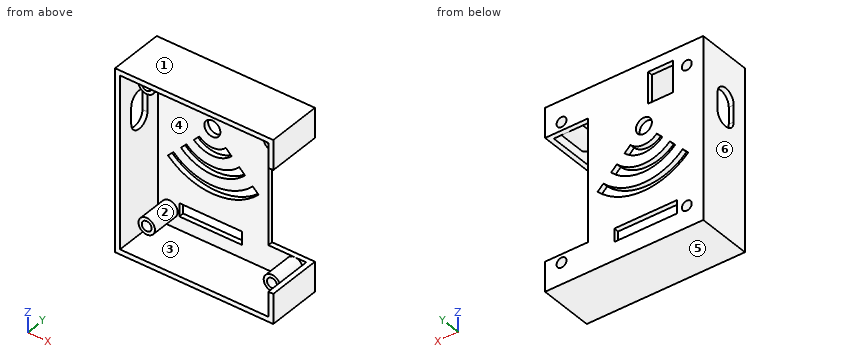
Autodesk Inventor part; units mm, degrees
ref_plane "YZ Plane" through (0, 0, 0) normal (1, 0, 0) x (0, 1, 0)
ref_plane "XZ Plane" through (0, 0, 0) normal (0, 1, 0) x (-1, 0, 0)
ref_plane "XY Plane" through (0, 0, 0) normal (0, 0, 1) x (1, 0, 0)
sketch "Sketch1" plane through (0, 0, 0) normal (0, 1, 0) x (-1, 0, 0)
  point P0 (0, 0)
sketch "Sketch2" plane through (0, 0, 0) normal (0, 1, 0) x (-1, 0, 0)
  line L0 (-24, 27.5) -> (24, 27.5)
  line L1 (24, 27.5) -> (24, -27.5)
  line L2 (24, -27.5) -> (-24, -27.5)
  line L3 (-24, -27.5) -> (-24, 27.5)
  line L4 (22.5, 26) -> (-22.5, 26)
  line L5 (-22.5, 26) -> (-22.5, -26)
  line L6 (-22.5, -26) -> (22.5, -26)
  line L7 (22.5, -26) -> (22.5, 26)
  dimension "d1" = 55
extrude "Extrusion1" add sketch "Sketch2" along normal blind 6
sketch "Sketch3" plane through (0, 6, 0) normal (0, 1, 0) x (1, 0, 0)
  circle A0 centre (19, -21) radius 2.5
  circle A1 centre (-19, -21) radius 2.5
  circle A2 centre (-19, 21) radius 2.5
  circle A3 centre (19, 21) radius 2.5
  circle A4 centre (-19, -21) radius 1.5
  circle A5 centre (-19, 21) radius 1.5
  circle A6 centre (19, 21) radius 1.5
  circle A7 centre (19, -21) radius 1.5
  line L0 (-22.5, -26) -> (22.5, -26)
  line L1 (22.5, -26) -> (22.5, 26)
  line L2 (22.5, 26) -> (-22.5, 26)
  line L3 (-22.5, 26) -> (-22.5, -26)
  line L4 (-24, -27.5) -> (24, -27.5)
  line L5 (24, -27.5) -> (24, 27.5)
  line L6 (24, 27.5) -> (-24, 27.5)
  line L7 (-24, 27.5) -> (-24, -27.5)
  dimension "d16" = 3
  dimension "d17" = 3
  dimension "d18" = 3
extrude "Extrusion2" add sketch "Sketch3" along normal blind 9
sketch "Sketch4" plane through (24, 0, 27.5) normal (1, 0, 0) x (0, 0, -1)
  line L0 (9, 6) -> (9, 15)
  line L1 (9, 15) -> (46, 15)
  line L2 (55, 0) -> (0, 0)
  line L3 (46, 6) -> (46, 15)
  line L4 (46, 15) -> (9, 15)
  line L5 (9, 15) -> (9, 6)
  line L6 (9, 0) -> (46, 0)
  line L7 (46, 0) -> (46, 15)
  line L8 (46, 15) -> (9, 15)
  line L9 (9, 15) -> (9, 0)
  point P0 (27.5, 0)
extrude "Extrusion3" cut sketch "Sketch4" against normal up to surface (1.5 mm away)
sketch "Sketch5" plane through (0, 15, 0) normal (0, 1, 0) x (1, 0, 0)
  line L0 (-24, -27.5) -> (24, -27.5)
  line L1 (-24, 27.5) -> (-24, -27.5)
  line L2 (24, -27.5) -> (-24, -27.5)
  line L3 (-24, -27.5) -> (-24, 27.5)
  line L4 (-24, 27.5) -> (24, 27.5)
  line L5 (22.5, -18.5) -> (24, -18.5)
  line L6 (24, -18.5) -> (11, -18.5)
  line L7 (24, 18.5) -> (24, 27.5)
  line L8 (24, 18.5) -> (11, 18.5)
  line L9 (11, 18.5) -> (11, -18.5)
  line L10 (24, 27.5) -> (24, 18.5)
  line L11 (24, -18.5) -> (24, -27.5)
  circle A0 centre (-19, -21) radius 1.5
  circle A1 centre (-19, -21) radius 1.5
  circle A2 centre (-19, 21) radius 1.5
  circle A3 centre (-19, 21) radius 1.5
  circle A4 centre (19, 21) radius 1.5
  circle A5 centre (19, 21) radius 1.5
  circle A6 centre (19, -21) radius 1.5
  circle A7 centre (19, -21) radius 1.5
  point P0 (0, 0)
extrude "Extrusion4" add sketch "Sketch5" along normal blind 1.5
sketch "Sketch6" plane through (-24, 0, -27.5) normal (-1, 0, 0) x (0, 0, 1)
  line L0 (41.4364, 10.844) -> (36.321, 10.844)
  line L1 (36.321, 4.444) -> (41.4364, 4.444)
  arc A0 (41.4364, 4.444) -> (41.4364, 10.844) centre (41.4364, 7.644) ccw
  arc A1 (36.321, 10.844) -> (36.321, 4.444) centre (36.321, 7.644) ccw
  point P0 (27.5, 0)
extrude "Extrusion5" cut sketch "Sketch6" against normal up to surface (1.5 mm away)
sketch "Sketch7" plane through (0, 16.5, 0) normal (0, 1, 0) x (1, 0, 0)
  circle A0 centre (-19, 21) radius 1.5
  line L0 (3, 18) -> (-16, 18)
  line L1 (-16, 18) -> (-16, 22)
  line L2 (-16, 22) -> (3, 22)
  line L3 (3, 22) -> (3, 18)
  point P0 (0, 0)
  dimension "d37" = 19
  dimension "d38" = 4
extrude "Extrusion6" cut sketch "Sketch7" against normal through all contours L0 L1 L2 L3
sketch "Sketch8" plane through (0, 16.5, 0) normal (0, 1, 0) x (1, 0, 0)
  line L0 (-14.75, -24.25) -> (-7.25, -24.25)
  line L1 (-7.25, -24.25) -> (-7.25, -14.75)
  line L2 (-7.25, -14.75) -> (-14.75, -14.75)
  line L3 (-14.75, -14.75) -> (-14.75, -24.25)
  point P0 (0, 0)
  dimension "d44" = 7.5
  dimension "d45" = 9.5
extrude "Extrusion7" cut sketch "Sketch8" against normal through all
sketch "Sketch9" plane through (0, 16.5, 0) normal (0, 1, 0) x (1, 0, 0)
  circle A0 centre (-5.9739, -8.7344) radius 2.43
  arc A1 (-1.887, -4.8042) -> (-9.9041, -4.6475) centre (-5.9739, -8.7344) ccw
  arc A2 (-0.1355, -3.1199) -> (-11.5884, -2.8959) centre (-5.9739, -8.7344) ccw
  arc A3 (2.1999, -0.874) -> (-13.8342, -0.5606) centre (-5.9739, -8.7344) ccw
  arc A4 (3.9514, 0.8103) -> (-15.5186, 1.1909) centre (-5.9739, -8.7344) ccw
  arc A5 (6.2868, 3.0561) -> (-17.7644, 3.5263) centre (-5.9739, -8.7344) ccw
  arc A6 (8.0389, 4.741) -> (-19.3203, 5.4014) centre (-5.9739, -8.7344) ccw
  line L0 (-19.3203, 5.4014) -> (-19.4487, 5.2778)
  line L1 (-19.4487, 5.2778) -> (-19.3445, 5.1695)
  line L2 (-17.7644, 3.5263) -> (-19.3445, 5.1695)
  line L3 (-13.8342, -0.5606) -> (-15.5186, 1.1909)
  line L4 (-9.9041, -4.6475) -> (-11.5884, -2.8959)
  line L5 (-1.887, -4.8042) -> (-0.1355, -3.1199)
  line L6 (2.1999, -0.874) -> (3.9514, 0.8103)
  line L7 (6.2868, 3.0561) -> (8.0389, 4.741)
  point P0 (0, 0)
  dimension "d48" = 4.86
extrude "Extrusion8" cut sketch "Sketch9" against normal through all
properties part number "Box2_Top"
Part model, mm, in its own coordinate system. Face numbers are marked on the shaded views. A direction names the side the tool comes from. Give positions to 0.01 mm unless a question says otherwise; leave off trailing zeros. Write each loop counter-clockwise with the first axis right and the second up, starting at its lowest first coordinate (ties: lowest second). Pieces come first, ordered by that corner, then holes. Notation, with made-up numbers: (83.25, 81.5) -> (126.25, 81.5) arc R29 ccw to (126.25, 106.5) -> close; hole circle Ø2 at (-9.75, 17.5). An arc over 180 degrees is marked (long way). Put each result on its own line as item: value. Start each with the question number.
Item 1: Cut at D-D (z = 8). List the corners of the cut face in (x, y).
Item 2: Pull direction Z, two halves, no side cores. Call the marked faces 3, 4, 5 and 6: pulls with the +Z half, pulls with the -Z half, needs draft (parallel to the pull), parting line crosses it, or undercut.
Item 3: Which spindle directions (+Z, -Z, +X, -X, +Y, -Y) get a long thin tool onto all of the face, cutting with end or side? Do the marked faces 1 and 2. Say none if no direction does.
Item 4: Cut at B-B (z = -21). List the corners of the cut face in (x, y).
Item 5: Cut at A-A (y = 13.25). State how many separate pieces and enclosed holes the cut face has, then the cut area to 3 significant figures.
Item 6: Pin check, flat tips, straight feed: pin 1 Ø5 at (x, z) = (-19, 21) entering from -Y; pin 2 Ø0.8 at (y, z) = (15.5, -1) entering from +X; pin 3 Ø22.5 at (x, z) = (7.5, 2.5) entering from -Y. Stop position of each tip, or through.
Item 7: Wall check: L1, parallel to Z at x = -19, y = 8; L2, parallel to X at y = 11, z = 21; L3, parallel to Z at x = -3, y = 11. Give the ranges that are in metal, low to high. Write a range as [from, to].
Item 8: Cut at C-C (x = -2.5). List the corners of the cut face in (y, z), then the cut area to 3 significant figures.
Answer list:
1. outline: (-24, 0) -> (-22.5, 0) -> (-22.5, 4.55) -> (-24, 4.55) -> close; (-24, 10.74) -> (-22.5, 10.74) -> (-22.5, 15) -> (-8.29, 15) -> (-8.29, 16.5) -> (-24, 16.5) -> close; (-3.66, 15) -> (11, 15) -> (11, 16.5) -> (-3.66, 16.5) -> close
2. face 3: undercut
2. face 4: undercut
2. face 5: pulls with the -Z half
2. face 6: needs draft
3. face 1: +Z, +X, -X, +Y, -Y
3. face 2: -Y
4. outline: (-24, 0) -> (-22.5, 0) -> (-22.5, 15) -> (-21.5, 15) -> (-21.5, 6) -> (-20.5, 6) -> (-20.5, 16.5) -> (-24, 16.5) -> close; (-17.5, 6) -> (-16.5, 6) -> (-16.5, 15) -> (-16, 15) -> (-16, 16.5) -> (-17.5, 16.5) -> close; (3, 15) -> (16.5, 15) -> (16.5, 6) -> (17.5, 6) -> (17.5, 16.5) -> (3, 16.5) -> close; (20.5, 6) -> (21.5, 6) -> (21.5, 15) -> (22.5, 15) -> (22.5, 0) -> (24, 0) -> (24, 16.5) -> (20.5, 16.5) -> close
5. separate pieces: 5
5. enclosed holes: 4
5. area: 295 mm2
6. pin 1: stops at y = 6
6. pin 2: stops at x = 11
6. pin 3: stops at y = 15
7. L1: z = [-27.5, -26], [-23.5, -22.5], [-19.5, -18.5], [18.5, 19.5], [22.5, 23.5], [26, 27.5]
7. L2: x = [-24, -22.5], [-21.5, -20.5], [-17.5, -16.5], [16.5, 17.5], [20.5, 21.5], [22.5, 24]
7. L3: z = [-27.5, -26], [26, 27.5]
8. outline: (0, -27.5) -> (16.5, -27.5) -> (16.5, -22) -> (15, -22) -> (15, -26) -> (0, -26) -> close; (0, 26) -> (15, 26) -> (15, 4.25) -> (16.5, 4.25) -> (16.5, 27.5) -> (0, 27.5) -> close; (15, -18) -> (16.5, -18) -> (16.5, -10.39) -> (15, -10.39) -> close; (15, -7.92) -> (16.5, -7.92) -> (16.5, -4.59) -> (15, -4.59) -> close; (15, -2.06) -> (16.5, -2.06) -> (16.5, 1.42) -> (15, 1.42) -> close
8. area: 110 mm2
